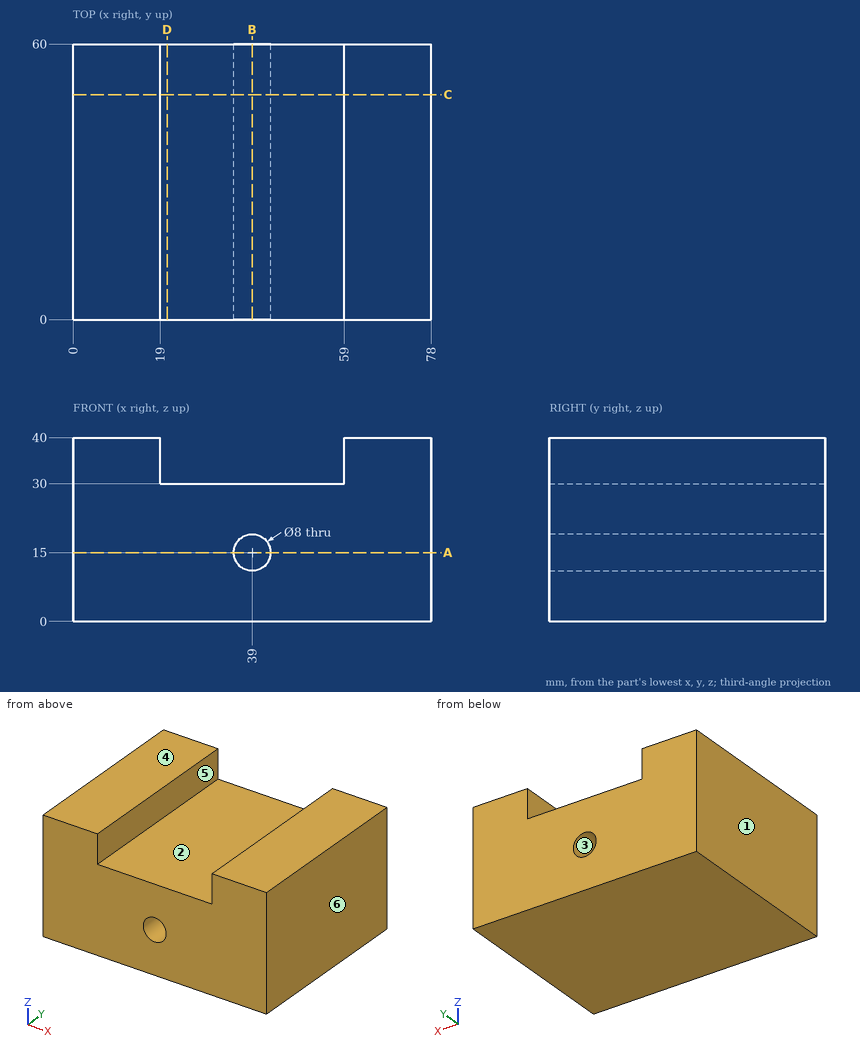
Study the drawing (mm; zero at the part's minimum x, y, z) and answer. A direction names the side the tool comes from. Round coordinates to 2 decimals unless told otherwise and drop trailing zeros. Write each loop counter-clockwise with the first axis right and the second up, starting at its lowest first coordinate (ties: lowest second). Pieces come first, ordered by that corner, then holes.
1) A cutting plane is placed at C-C on y = 49. Determine the outline of the cut face in (x, z).
2) Determine the mould class of the marked faces 3, 4, 5 and 6 for opening direction X: pulls with the +X half, pulls with the -X half, needs draft (parallel to the pull), parting line crosses it, or undercut.
3) A flat-ended cylindrical pin translates along its axis: P1, Ø1, axis at x = 48.5, y = 34, coming from the +Z side. Find the tip coordinate at first contact, or state that the pin passes through.
4) A cutting plane is placed at D-D on x = 20.5. Determine the outline of the cut face in (y, z).
5) Which of the six approach directions +Z, -Z, +X, -X, +Y, -Y give full straight-line access (tool end or side, diameter ignored) to the marked faces 1 and 2?
6) A cutting plane is placed at B-B on x = 39. Determine the outline of the cut face in (y, z).
7) A cutting plane is placed at A-A on z = 15. Determine the outline of the cut face in (x, y), and give its area (3 significant figures).
8) Consider probe 1 along X at (y, z) = (12.5, 15); probe 2 along X at (y, z) = (50, 34); probe 3 along Z at (x, y) = (38.5, 38). Determine where each line is inside the solid, lowest interval first.
Entries:
1. outline: (0, 0) - (78, 0) - (78, 40) - (59, 40) - (59, 30) - (19, 30) - (19, 40) - (0, 40) - close; hole circle Ø8 at (39, 15)
2. face 3: undercut
2. face 4: needs draft
2. face 5: undercut
2. face 6: pulls with the +X half
3. P1: stops at z = 30
4. outline: (0, 0) - (60, 0) - (60, 30) - (0, 30) - close
5. face 1: +Z, -Z, -X, +Y, -Y
5. face 2: +Z, +Y, -Y
6. outline: (0, 0) - (60, 0) - (60, 11) - (0, 11) - close; (0, 19) - (60, 19) - (60, 30) - (0, 30) - close
7. outline: (0, 0) - (35, 0) - (35, 60) - (0, 60) - close; (43, 0) - (78, 0) - (78, 60) - (43, 60) - close
7. area: 4,200 mm2
8. probe 1: x = 0 to 35, 43 to 78
8. probe 2: x = 0 to 19, 59 to 78
8. probe 3: z = 0 to 11.03, 18.97 to 30
